Drawing for the job (mm, zero at the part's lowest x, y, z). A direction names the side the tool comes from. Give positions to 0.01 mm unless a question says otherwise; leave off trailing zeros. Order: outer loops, then holes, each group sorted by start corner. A loop starts at its lowest first (then second) coordinate and runs counter-clockwise, first axis right, second up. Notation, with made-up numbers: M 60.25,-20 L 96.25,-20 A13 cw 96.25,-8 Z; hole C -36.75,6.25 d6. An arc over 180 degrees is marked long. One line per item, written item: value.
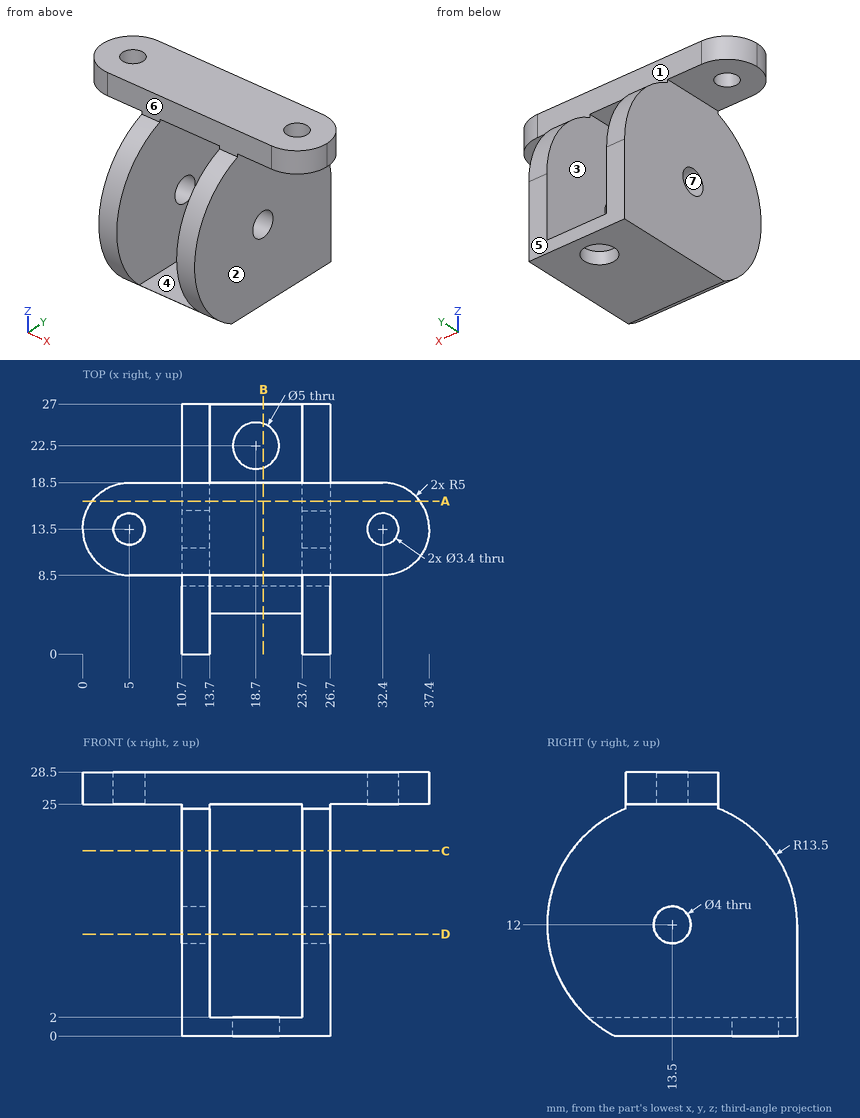
1) Pin check, flat tips, straight feed: pin 1 (2.5 mm diameter, centred on x = 32.4, y = 13.5, fed in from +Z); pin 2 (11.5 mm diameter, centred on y = 19.5, z = 10.5, fed in from +X); pin 3 (2 mm diameter, centred on x = 20, z = 27.5, fed in from -Y); pin 4 (4.5 mm diameter, centred on y = 13.5, z = 12, fed in from -X). Stop position of each tip, or through.
Check values:
pin 1: through
pin 2: x = 26.7
pin 3: y = 8.5
pin 4: x = 10.7
2) Saw through at A-A, the plane y = 16.5. Write the cut outline in (x, z).
Check values:
outline: M 1,25 L 10.7,25 L 10.7,0 L 26.7,0 L 26.7,25 L 36.4,25 L 36.4,28.5 L 1,28.5 Z; hole M 13.7,2 L 23.7,2 L 23.7,25 L 13.7,25 Z
3) Saw through at C-C, the plane z = 20. Write the cut outline in (x, y).
Check values:
outline: M 10.7,2.63 L 13.7,2.63 L 13.7,24.37 L 10.7,24.37 Z; M 23.7,2.63 L 26.7,2.63 L 26.7,24.37 L 23.7,24.37 Z
4) Tool access for the marked faces 1, 2 and 3: list every direction of +Z, -Z, +X, -X, +Y, -Y with a clear straight run to the whole face (end or side of a thin tool).
Check values:
face 1: +Z, +X, -X, +Y
face 2: -Z, +X, +Y, -Y
face 3: +Y, -Y
5) Drill centre lines: probe 1 along X at (y, z) = (16, 20.25); probe 2 along Z at (x, y) = (24.5, 12); probe 3 along Z at (x, y) = (7.5, 8.75). Where is each one in solid material? Low to high. Write a range as from..to.
Check values:
probe 1: 10.7..13.7, 23.7..26.7
probe 2: 0..10.68, 13.32..28.5
probe 3: 25..28.5
6) Saw through at D-D, the plane z = 11. Write the cut outline in (x, y).
Check values:
outline: M 10.7,0.04 L 13.7,0.04 L 13.7,11.77 L 10.7,11.77 Z; M 10.7,15.23 L 13.7,15.23 L 13.7,27 L 10.7,27 Z; M 23.7,0.04 L 26.7,0.04 L 26.7,11.77 L 23.7,11.77 Z; M 23.7,15.23 L 26.7,15.23 L 26.7,27 L 23.7,27 Z
7) Mould opens along Y. For the marked faces 4, 5, 6 and 7 say: released by +Y, released by -Y, zero draft, split by the parting line, or undercut.
Check values:
face 4: zero draft
face 5: released by +Y
face 6: released by -Y
face 7: undercut
8) Saw through at B-B, the plane x = 19.5. Write the cut outline in (y, z).
Check values:
outline: M 4.43,2 A13.5 ccw 7.32,0 L 20.13,0 L 20.13,2 Z; M 8.5,25 L 18.5,25 L 18.5,28.5 L 8.5,28.5 Z; M 24.87,0 L 27,0 L 27,2 L 24.87,2 Z
